Job drawing, mm, ordinate dimensions from the low corner. One solid piece. A direction names the side the tool comes from. Coordinates: 2 decimals unless noted, no trailing zeros. Write each loop counter-clockwise with the first axis right and the second up, starting at its lowest first coordinate (ties: lowest second). Pieces come first, ordered by that corner, then holes. Notation, with made-up numbers: (46, -32.75) -> (62, -32.75) arc R26 ccw to (62, 0.25) -> close; hole circle Ø11 at (-24, 82). An arc over 180 degrees is marked (long way). Answer as a JSON object with one key per item and string values. Group by question number.
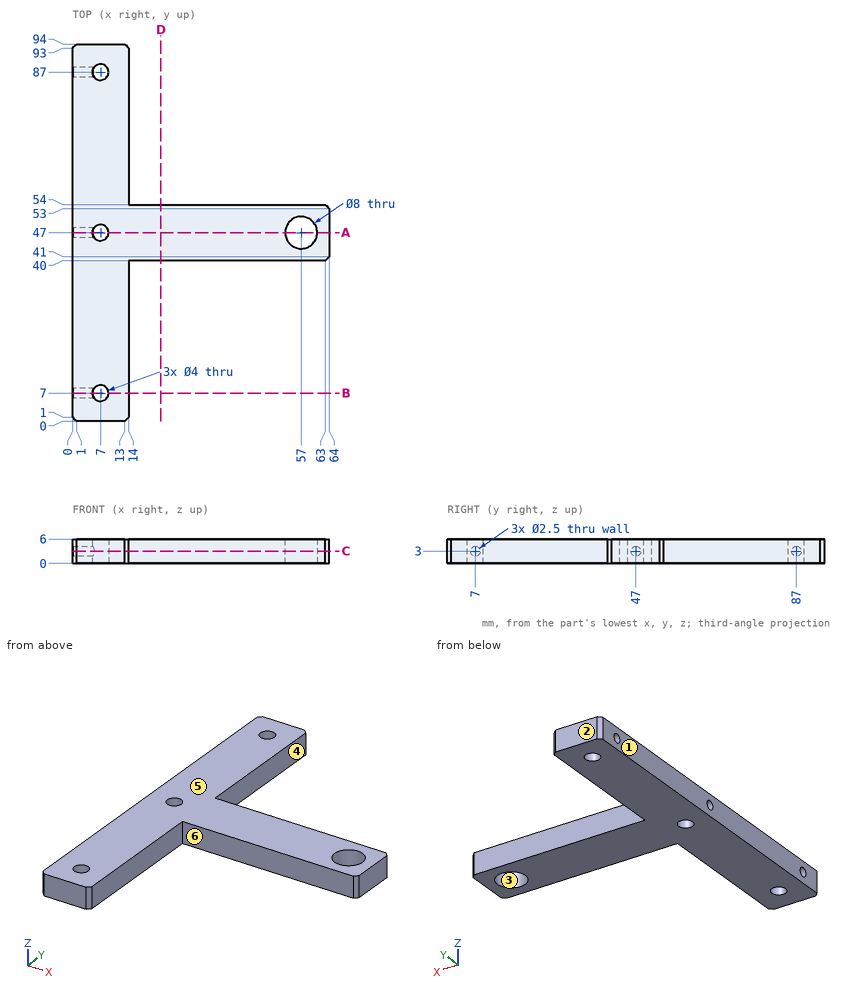
(1) Cut at B-B on y = 7. List the corners of the cut face in (x, z), plus the area to 3 significant figures.
(2) Cut at D-D on x = 22. List the corners of the cut face in (y, z), plus the area to 3 significant figures.
(3) Cut at C-C on z = 3. List the corners of the cut face in (x, y), plus the area to 3 significant figures.
(4) Pin check, flat tips, straight feed: pin 1 (1.5 mm diameter, centred on x = 27.5, z = 5.5, fed in from +Y); pin 2 (2 mm diameter, centred on y = 87, z = 3, fed in from -X); pin 3 (1.5 mm diameter, centred on x = 12, z = 5.5, fed in from -Y); pin 4 (3 mm diameter, centred on y = 82.5, z = 3.5, fed in from +X). Stop position of each tip, or through.
(5) Wall check: probe 1 along Y at (x, z) = (1.9, 3); probe 2 along Y at (x, z) = (7, 1.5); probe 3 along X at (y, z) = (87, 4.75). Give the ranges that are in metal, low to high.
(6) Pull direction X, two halves, no side cores. Call the marked faces 1, 2 and 3: released by +X, released by -X, zero draft, split by the parting line, or undercut.
(7) 3-axis set-ups, long thin cutter, end or side, ignore diameter. For the marked faces 4, 5 and 6: which of +Z, -Z, +X, -X, +Y, -Y reach the whole face in a straight line?
(8) Cut at A-A on y = 47. List the corners of the cut face in (x, z), plus the area to 4 significant figures.
Results found:
{
 "1": {"outline": "(0, 0) -> (5, 0) -> (5, 1.75) -> (0, 1.75) -> close; (0, 4.25) -> (5, 4.25) -> (5, 6) -> (0, 6) -> close; (9, 0) -> (14, 0) -> (14, 6) -> (9, 6) -> close", "area": "47.5 mm²"},
 "2": {"outline": "(40, 0) -> (54, 0) -> (54, 6) -> (40, 6) -> close", "area": "84.0 mm²"},
 "3": {"outline": "(0, 1) -> (1, 0) -> (13, 0) -> (14, 1) -> (14, 40) -> (63, 40) -> (64, 41) -> (64, 53) -> (63, 54) -> (14, 54) -> (14, 93) -> (13, 94) -> (1, 94) -> (0, 93) -> (0, 88.25) -> (5.44, 88.25) arc R2 cw (long way) to (5.44, 85.75) -> (0, 85.75) -> (0, 48.25) -> (5.44, 48.25) arc R2 cw (long way) to (5.44, 45.75) -> (0, 45.75) -> (0, 8.25) -> (5.44, 8.25) arc R2 cw (long way) to (5.44, 5.75) -> (0, 5.75) -> close; hole circle Ø8 at (57, 47)", "area": "1,890 mm²"},
 "4": {"pin 1": "stops at y = 54", "pin 2": "stops at x = 8.73", "pin 3": "stops at y = 0", "pin 4": "stops at x = 14"},
 "5": {"probe 1": "y = 0 to 5.75, 8.25 to 45.75, 48.25 to 85.75, 88.25 to 94", "probe 2": "y = 0 to 5, 9 to 45, 49 to 85, 89 to 94", "probe 3": "x = 0 to 5, 9 to 14"},
 "6": {"face 1": "released by -X", "face 2": "zero draft", "face 3": "undercut"},
 "7": {"face 4": "+Z, -Z, +X, +Y", "face 5": "+Z, +X, -X, +Y, -Y", "face 6": "+Z, -Z, +X, -Y"},
 "8": {"outline": "(0, 0) -> (5, 0) -> (5, 1.75) -> (0, 1.75) -> close; (0, 4.25) -> (5, 4.25) -> (5, 6) -> (0, 6) -> close; (9, 0) -> (53, 0) -> (53, 6) -> (9, 6) -> close; (61, 0) -> (64, 0) -> (64, 6) -> (61, 6) -> close", "area": "299.5 mm²"}
}
